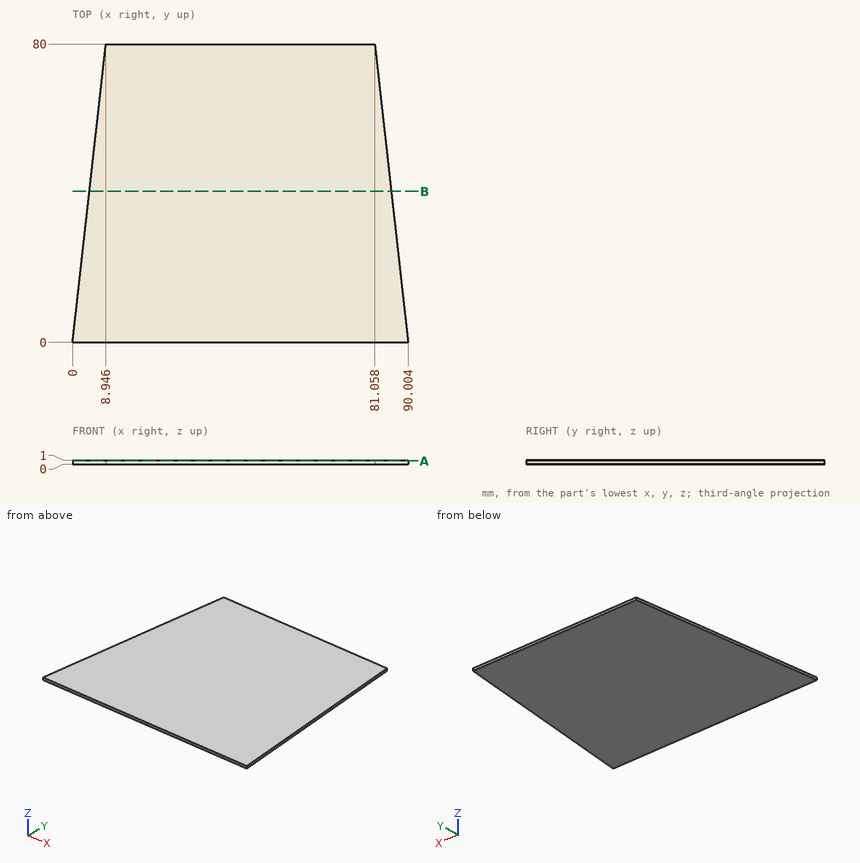
Geometry check sheet. Reference: drawing and pictorial views, mm from the part's lowest x, y, z. Coordinates: 2 decimals unless noted, no trailing zeros. Write each loop counter-clockwise with the first axis right and the second up, starting at its lowest first coordinate (ties: lowest second). Pieces come first, ordered by that corner, then holes. Notation, with made-up numbers: M -18.5,59 L -6.5,59 A20 ccw -6.5,90 Z; hole C 89,33 d9. An arc over 180 degrees is marked long. Use one line per item in the form item = value.
Item 1: Sectioned sample at B-B, the plane y = 40.5. Record the cut outline in (x, z) (3 decimals).
Answer below:
outline = M 4.529,0 L 85.475,0 L 85.475,1 L 4.529,1 Z
Item 2: Sectioned sample at A-A, the plane z = 0.85. Record the cut outline in (x, y), and give its area (3 significant figures).
Answer below:
outline = M 0,0 L 90,0 L 81.06,80 L 8.95,80 Z
area = 6,480 mm^2
Item 3: Gauge pin test, flat end, axial feed: pin 1 Ø3 at (x, y) = (78.5, 14.5) entering from -Z. Record the tip position at first contact, or that the pin passes through.
Answer below:
pin_1 = 0
Item 4: Material ranges on L1, parallel to X at y = 67.5, z = 0.75; L2, parallel to X at y = 70, z = 0.3, recorded low to high. Write a range as from..to.
Answer below:
L1 = 7.55..82.46
L2 = 7.83..82.18
